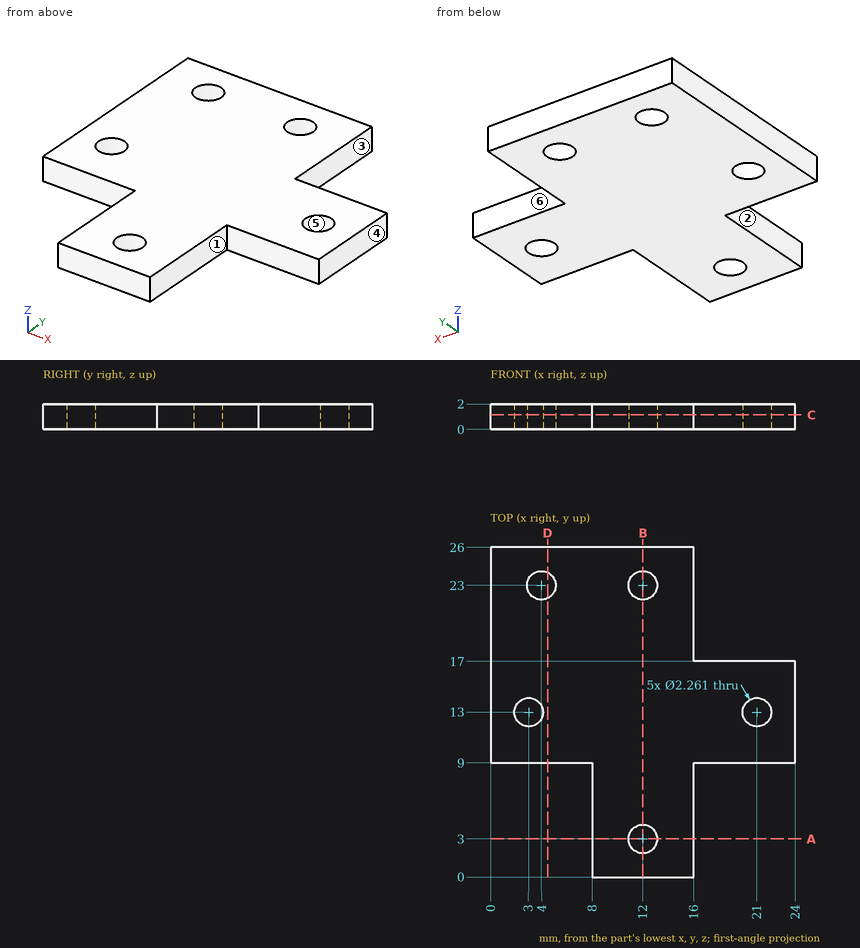
Print and shaded views of the part. All mm, measured from the part's lowest x, y and z. A direction names the side the tool comes from. Round coordinates to 2 decimals unless told otherwise and drop trailing zeros. Order: outer loops, then holes, each group sorted by start corner. A loop starts at its lowest first (then second) coordinate and runs counter-clockwise, first axis right, second up.
Q1. Wall check: L1, parallel to Y at x = 12, z = 1.6; L2, parallel to Y at x = 21, z = 0.7; L3, parallel to X at y = 23.25, z = 0.7. Give the ranges that are in metal, low to high.
Q2. Drop flat-ended pins along their axis: pin 1 (6 mm diameter, centred on x = 13, y = 23, fed in from -Z); pin 2 (1.8 mm diameter, centred on x = 12, y = 23, fed in from +Z); pin 3 (1 mm diameter, centred on x = 20.5, z = 1.5, fed in from +Y); pin 4 (1 mm diameter, centred on y = 5.5, z = 0.5, fed in from -X). Give the stop position or say it passes through.
Q3. Slice it at A-A (y = 3). Write the cut outline in (x, z).
Q4. Slice it at D-D (x = 4.5). Write the cut outline in (y, z).
Q5. Slice it at B-B (x = 12). Write the cut outline in (y, z).
Q6. Which spindle directions (+Z, -Z, +X, -X, +Y, -Y) get a long thin tool onto all of the face, cutting with end or side? Do the marked faces 1, 2 and 3. Say none if no direction does.
Q7. Slice it at C-C (z = 1.15). Write the cut outline in (x, y), and give its area (3 significant figures).
Q8. Two-plate mould, pull along X, no slides. Class the marked faces 4, 5 and 6: pulls with the +X half, pulls with the -X half, needs draft (parallel to the pull), parting line crosses it, or undercut.
Results below:
1. L1: y = 0 to 1.87, 4.13 to 21.87, 24.13 to 26
1. L2: y = 9 to 11.87, 14.13 to 17
1. L3: x = 0 to 2.9, 5.1 to 10.9, 13.1 to 16
2. pin 1: stops at z = 0
2. pin 2: passes through
2. pin 3: stops at y = 17
2. pin 4: stops at x = 8
3. outline: (8, 0) - (10.87, 0) - (10.87, 2) - (8, 2) - close; (13.13, 0) - (16, 0) - (16, 2) - (13.13, 2) - close
4. outline: (9, 0) - (21.99, 0) - (21.99, 2) - (9, 2) - close; (24.01, 0) - (26, 0) - (26, 2) - (24.01, 2) - close
5. outline: (0, 0) - (1.87, 0) - (1.87, 2) - (0, 2) - close; (4.13, 0) - (21.87, 0) - (21.87, 2) - (4.13, 2) - close; (24.13, 0) - (26, 0) - (26, 2) - (24.13, 2) - close
6. face 1: +Z, -Z, +X, -Y
6. face 2: +Z, -Z, -X, -Y
6. face 3: +Z, -Z, +X, +Y
7. outline: (0, 9) - (8, 9) - (8, 0) - (16, 0) - (16, 9) - (24, 9) - (24, 17) - (16, 17) - (16, 26) - (0, 26) - close; hole circle Ø2.26 at (3, 13); hole circle Ø2.26 at (4, 23); hole circle Ø2.26 at (12, 3); hole circle Ø2.26 at (12, 23); hole circle Ø2.26 at (21, 13)
7. area: 388 mm2
8. face 4: pulls with the +X half
8. face 5: undercut
8. face 6: needs draft
